Geometry: final body of the model. Coordinates: model frame, mm. A direction names the side the tool comes from. Round coordinates to 2 decimals unless told otherwise and drop trailing zeros. Loops run counter-clockwise (first coordinate to the right, second up) from the corner with the lowest first, then second, coordinate; pieces in that order, holes last. Notation, with made-up numbers: M 55,71 L 94,71 A25 cw 94,107 Z; hole C 39,25.25 d9. An arc over 180 degrees is marked long. Return JSON: item names as keys, results as strings.
Autodesk Inventor part; units mm, degrees
ref_plane "YZ Plane" through (0, 0, 0) normal (1, 0, 0) x (0, 1, 0)
ref_plane "XZ Plane" through (0, 0, 0) normal (0, 1, 0) x (-1, 0, 0)
ref_plane "XY Plane" through (0, 0, 0) normal (0, 0, 1) x (1, 0, 0)
sketch "Sketch1" plane through (0, 0, 0) normal (0, 1, 0) x (-1, 0, 0)
  circle A0 centre (0, 0) radius 25
  dimension "d0" = 50
extrude "Extrusion1" add sketch "Sketch1" along normal blind 250
sketch "Sketch2" plane through (0, 250, 0) normal (0, 1, 0) x (1, 0, 0)
  circle A0 centre (0, 0) radius 25
  dimension "d3" = 50
extrude "Extrusion2" cut sketch "Sketch2" against normal blind 10
sketch "Sketch3" plane through (0, 240, 0) normal (0, 1, 0) x (1, 0, 0)
  circle A0 centre (0, 0) radius 22.5
  dimension "d6" = 45
extrude "Extrusion3" add sketch "Sketch3" along normal blind 10
sketch "Sketch4" plane through (0, 0, 0) normal (0, -1, 0) x (1, 0, 0)
  circle A0 centre (0, 0) radius 25
  dimension "d9" = 50
extrude "Extrusion4" cut sketch "Sketch4" against normal blind 50
sketch "Sketch5" plane through (0, 50, 0) normal (0, -1, 0) x (1, 0, 0)
  circle A0 centre (0, 0) radius 50
  dimension "d12" = 100
extrude "Extrusion5" add sketch "Sketch5" against normal blind 30
properties part number "expo1"
Q1. Section query A-A (z = 0). Output: boundary loops of the cut face in (x, y), plus the area to 4 significant figures.
Determined:
{"outline": "M -50,50 L 50,50 L 50,80 L 25,80 L 25,240 L 22.5,240 L 22.5,250 L -22.5,250 L -22.5,240 L -25,240 L -25,80 L -50,80 Z", "area": "11,450 mm^2"}
Q2. Reachability of faces 1 (the flat face through (0, 250, 0)), 2 (the flat face through (-22.9, 80, -10.4)) from +Z, -Z, +X, -X, +Y, -Y: full face, straight path, thin tool, end or side. Return the list, or none.
Determined:
{"face 1": "+Z, -Z, +X, -X, +Y", "face 2": "+Y"}
Q3. Material intervals for L1, parallel to Z at x = -0.5, y = 102 (3 decimals); L2, parallel to Y at x = 35, z = 0; L3, parallel to X at y = 168, z = -1.5, sorted ascending.
Determined:
{"L1": "z = -24.995 to 24.995", "L2": "y = 50 to 80", "L3": "x = -24.95 to 24.95"}
Q4. Section query D-D (y = 78). Output: boundary loops of the cut face in (x, z).
Determined:
{"outline": "C 0,0 d100"}
Q5. Pin query (flat end, axial travel): pin 1 (3 mm diameter, centred on y = 74, z = -32, fed in from -X); pin 2 (1.5 mm diameter, centred on x = 35.5, y = 79, fed in from +Z); pin 3 (2 mm diameter, centred on y = 177.5, z = -20, fed in from -X). Return the tip coordinate at first contact, or that it passes through.
Determined:
{"pin 1": "stops at x = -39.62", "pin 2": "stops at z = 35.95", "pin 3": "stops at x = -16.25"}
Q6. Section query B-B (x = 0). Output: boundary loops of the cut face in (y, z).
Determined:
{"outline": "M 50,-50 L 80,-50 L 80,-25 L 240,-25 L 240,-22.5 L 250,-22.5 L 250,22.5 L 240,22.5 L 240,25 L 80,25 L 80,50 L 50,50 Z"}
Q7. Section query C-C (y = 107). Output: boundary loops of the cut face in (x, z), plus the area to 3 significant figures.
Determined:
{"outline": "C 0,0 d50", "area": "1,960 mm^2"}
